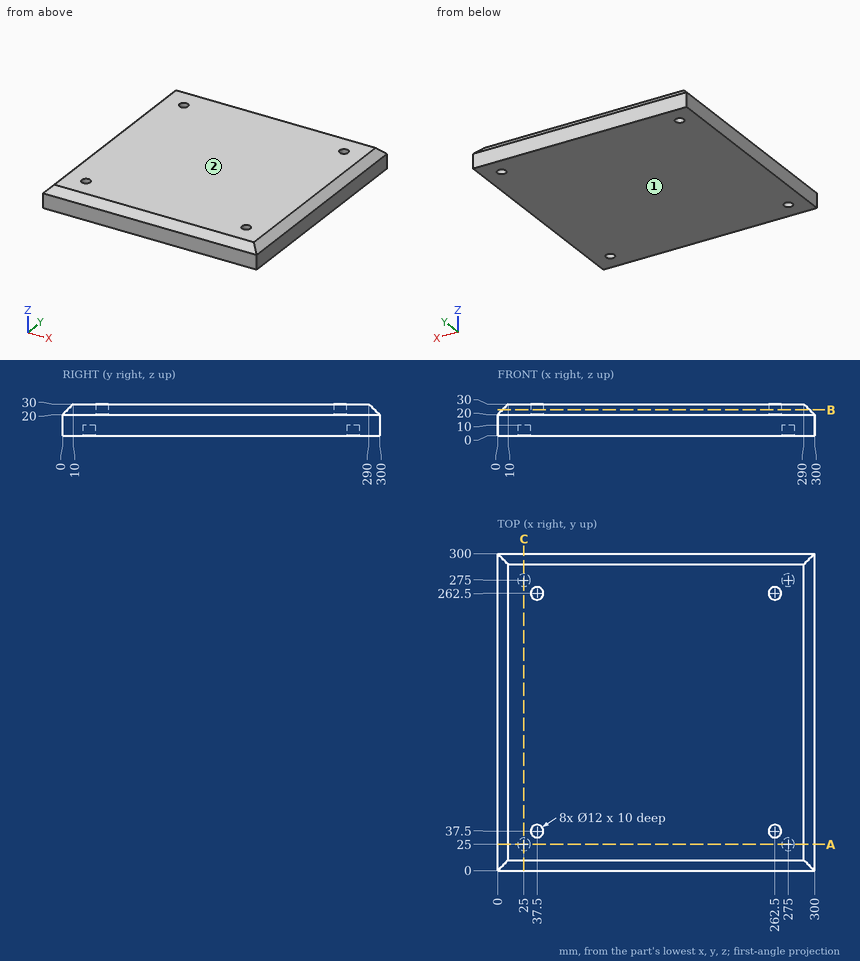
Here's the drawing with two shaded views (mm, measured from the low corner). I have some questions. Round coordinates to 2 decimals unless told otherwise and drop trailing zeros. Order: outer loops, then holes, each group sorted by start corner. A loop starts at its lowest first (then second) coordinate and runs counter-clockwise, first axis right, second up. Notation, with made-up numbers: (73, -1) -> (131, -1) arc R22 ccw to (131, 22) -> close; hole circle Ø10 at (-5.5, -25.75). An arc over 180 degrees is marked (long way). Write each question's results on one line, items separated by ' | '. Start each with the question number.
Item 1: If we section it at B-B, the plane z = 24.5: Write out the boundary of the cut face in (x, y), then the cut area to 3 significant figures.
Item 2: Will these pins go through, and if not, where does the flat tip stop? pin 1 (6 mm diameter, centred on x = 116, z = 27, fed in from -Y); pin 2 (3.5 mm diameter, centred on x = 263, y = 261, fed in from +Z); pin 3 (13 mm diameter, centred on x = 35, y = 262, fed in from +Z); pin 4 (11 mm diameter, centred on x = 275, y = 275, fed in from -Z).
Item 3: Thinking about a two-plate mould opening in Z: for the marked faces 1 and 2, which applies, +Z half, -Z half, draft (parallel to the pull), parting line (faces both ways), or undercut?
Item 4: Please list where these lines run through material, in increasing order: L1, parallel to Y at x = 262.5, z = 22.5; L2, parallel to Y at x = 37.5, z = 24.25; L3, parallel to Y at x = 187, z = 26.
Item 5: If we section it at A-A, the plane y = 25: Write out the boundary of the cut face in (x, z), then the cut area to 3 significant figures.
Results:
1) outline: (4.5, 4.5) -> (295.5, 4.5) -> (295.5, 295.5) -> (4.5, 295.5) -> close; hole circle Ø12 at (37.5, 37.5); hole circle Ø12 at (37.5, 262.5); hole circle Ø12 at (262.5, 37.5); hole circle Ø12 at (262.5, 262.5) | area: 84,200 mm2
2) pin 1: stops at y = 4 | pin 2: stops at z = 20 | pin 3: stops at z = 30 | pin 4: stops at z = 10
3) face 1: -Z half | face 2: +Z half
4) L1: y = 2.5 to 31.5, 43.5 to 256.5, 268.5 to 297.5 | L2: y = 4.25 to 31.5, 43.5 to 256.5, 268.5 to 295.75 | L3: y = 6 to 294
5) outline: (0, 0) -> (19, 0) -> (19, 10) -> (31, 10) -> (31, 0) -> (269, 0) -> (269, 10) -> (281, 10) -> (281, 0) -> (300, 0) -> (300, 20) -> (290, 30) -> (10, 30) -> (0, 20) -> close | area: 8,660 mm2
